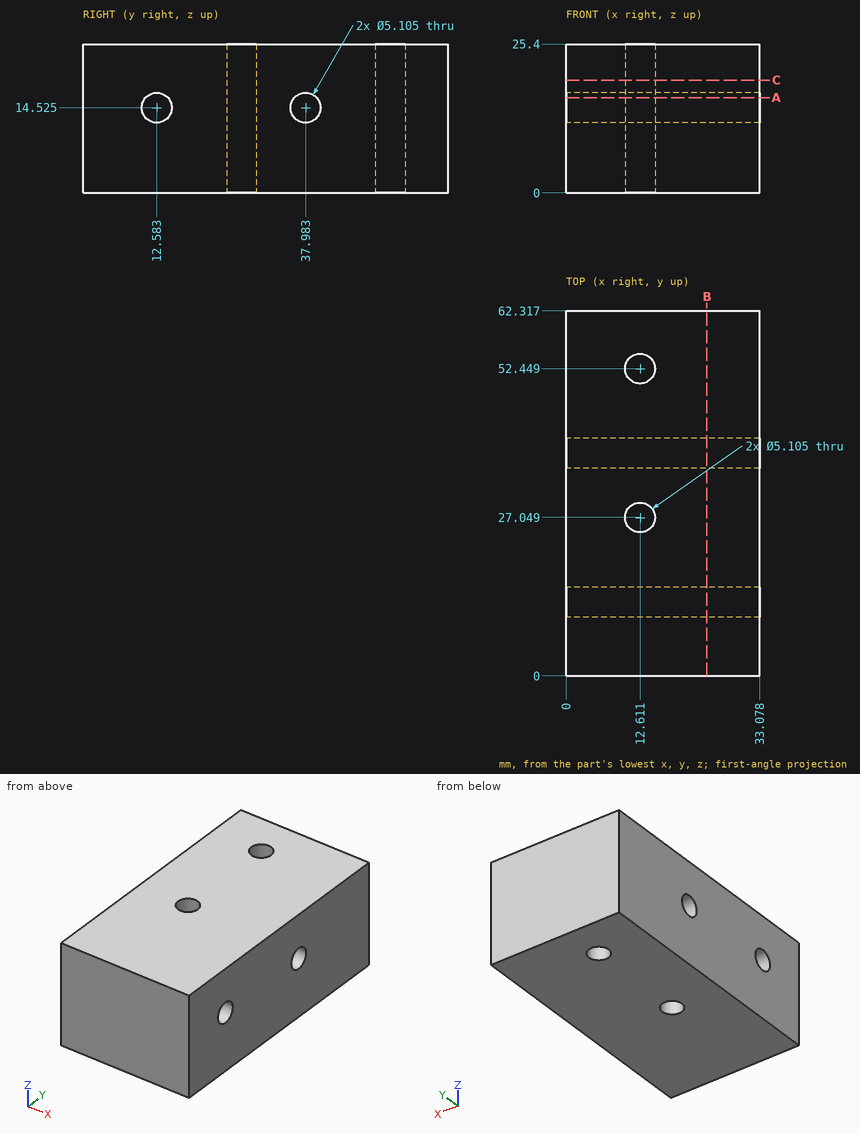
Geometry check sheet. Reference: drawing and pictorial views, mm from the part's lowest x, y, z. Round coordinates to 2 decimals unless told otherwise and drop trailing zeros. Order: outer loops, then holes, each group sorted by start corner. A loop starts at its lowest first (then second) coordinate and runs counter-clockwise, first axis right, second up. Notation, with made-up numbers: (75, 7.5) - (110, 7.5) arc R23 cw to (110, 15.5) - close; hole circle Ø8 at (45, -38.5). An arc over 180 degrees is marked (long way). One line per question, with ' | ' between items. Start each with the question number.
(1) Thickness scan on L1, parallel to Z at x = 29, y = 38; L2, parallel to Y at x = 21, z = 13 (1 decimal); L3, parallel to Y at x = 11, z = 8.25 (1 decimal). Record the ranges inside material, lowest first. Write a range as [from, to].
(2) Sectioned sample at A-A on z = 16.25. Record the cut outline in (x, y) (1 decimal).
(3) Depth check by flat-ended pin: pin 1 Ø8 at (x, y) = (8, 33) entering from -Z. Enter the tip coordinate at first touch or a pass-through.
(4) Sectioned sample at B-B on x = 24. Record the cut outline in (y, z) (1 decimal), and give its area (3 significant figures).
(5) Sectioned sample at C-C on z = 19.25. Record the cut outline in (x, y) (1 decimal), and give its area (3 significant figures).
Conclusion:
1) L1: z = [0, 11.97], [17.08, 25.4] | L2: y = [0, 10.5], [14.6, 35.9], [40, 62.3] | L3: y = [0, 25.1], [29, 50.5], [54.4, 62.3]
2) outline: (0, 0) - (33.1, 0) - (33.1, 10.7) - (0, 10.7) - close; (0, 14.5) - (33.1, 14.5) - (33.1, 36.1) - (0, 36.1) - close; (0, 39.9) - (33.1, 39.9) - (33.1, 62.3) - (0, 62.3) - close; hole circle Ø5.1 at (12.6, 27); hole circle Ø5.1 at (12.6, 52.4)
3) pin 1: stops at z = 0
4) outline: (0, 0) - (62.3, 0) - (62.3, 25.4) - (0, 25.4) - close; hole circle Ø5.1 at (12.6, 14.5); hole circle Ø5.1 at (38, 14.5) | area: 1,540 mm2
5) outline: (0, 0) - (33.1, 0) - (33.1, 62.3) - (0, 62.3) - close; hole circle Ø5.1 at (12.6, 27); hole circle Ø5.1 at (12.6, 52.4) | area: 2,020 mm2
